Autodesk Inventor part; units mm, degrees
ref_plane "YZ Plane" through (0, 0, 0) normal (1, 0, 0) x (0, 1, 0)
ref_plane "XZ Plane" through (0, 0, 0) normal (0, 1, 0) x (-1, 0, 0)
ref_plane "XY Plane" through (0, 0, 0) normal (0, 0, 1) x (1, 0, 0)
sketch "Skizze3" plane through (0, 0, 0) normal (0, 0, 1) x (1, 0, 0)
  line L0 (0, 0) -> (-80, 0)
  line L1 (-80, 0) -> (-80, 100)
  line L2 (-80, 100) -> (0, 100)
  line L3 (0, 100) -> (0, 0)
  line L4 (-80, 100) -> (0, 100)
  line L5 (-40, 105.85) -> (-80, 105.85)
  line L6 (-80, 105.85) -> (-80, 100)
  line L7 (-80, 50) -> (-85.85, 50)
  line L8 (-85.85, 50) -> (-85.85, 98.2)
  line L9 (-85.85, 98.2) -> (-80, 98.2)
  line L10 (-80, 98.2) -> (-80, 50)
  line L11 (-40, 105.85) -> (-40, 100)
  dimension "d4" = 100
  dimension "d5" = 80
  dimension "d6" = 5.85
  dimension "d7" = 5.85
  dimension "d8" = 1.8
extrude "Extrusion3" add sketch "Skizze3" along normal blind 5 contours L0 L1 L2 L3
extrude "Extrusion4" add sketch "Skizze3" along normal blind 5 contours L7 L8 L9 L1 | L2 L6 L5 L11
fillet "Rundung1" radius 2 2 edges at (-85.85, 98.2, 2.5) (-80, 105.85, 2.5)
mirror "Spiegeln1" about plane through (-85.85, 50, 0) normal (0, -1, 0) of "Extrusion4", "Rundung1"
mirror "Spiegeln2" about plane through (-40, 0, 0) normal (1, 0, 0) of "Extrusion4", "Rundung1", "Spiegeln1"
fillet "Rundung2" radius 1.5 4 edges at (-80, 98.2, 2.5) (-80, 1.8, 2.5) (0, 1.8, 2.5) (0, 98.2, 2.5)
sketch "Skizze4" plane through (0, 0, 5) normal (0, 0, 1) x (1, 0, 0)
  circle A0 centre (-66.2696, 23.5053) radius 7.471
  point P0 (0, 0)
  point P1 (-74.5257, 11.4963)
  point P2 (-75.2763, 39.7173)
  point P3 (-61.9163, 37.7659)
  point P4 (-59.3644, 15.2491)
extrude "Extrusion5" cut sketch "Skizze4" against normal blind 10
equation "\"d7\" = d6"
properties part number "BT701_trajan20_21" material "Acryl"
CAD build for the part. Positions are in the model's coordinates, mm. A direction names the side the tool comes from. Round coordinates to 2 decimals unless told otherwise and drop trailing zeros. Write each loop counter-clockwise with the first axis right and the second up, starting at its lowest first coordinate (ties: lowest second). Pieces come first, ordered by that corner, then holes. Notation, with made-up numbers: (88.25, -34.5) -> (144.25, -34.5) arc R14 ccw to (144.25, -10.5) -> close; hole circle Ø4 at (-16.5, -5). An arc over 180 degrees is marked (long way). Answer in a Markdown table with one row per item. Add a question column.
Item 1: Drill centre lines: line 1 (X direction, y = 20.5, z = 2.65); line 2 (X direction, y = 20, z = 2.6); line 3 (X direction, y = 0.5, z = 1.75). Where is each one in solid material? Low to high. Write a range as from..to.
Item 2: Saw through at A-A, the plane z = 3.2. Write the cut outline in (x, y).
Item 3: Which spindle directions (+Z, -Z, +X, -X, +Y, -Y) get a long thin tool onto all of the face, cutting with end or side? Do faces 1 (the face through (0, -2, 2)), 2 (the face through (-83, 98.2, 2)), 3 (the face through (-41, -5.85, 2)), 4 (the face through (0, 102, 2)), 5 (the face through (-83, 1.8, 2)). Say none if no direction does.
Item 4: Drop flat-ended pins along their axis: pin 1 Ø2 at (y, z) = (101, 2.5) entering from +X; pin 2 Ø2 at (y, z) = (-2, 3) entering from -X; pin 3 Ø2.5 at (x, z) = (2, 1.5) entering from -Y; pin 4 Ø3 at (x, y) = (-22.5, 28) entering from -Z. Give the stop position or say it passes through.
Findings below:
| question | item | result |
|---|---|---|
| 1 | line 1 | x = -85.85..-73.11, -59.43..5.85 |
| 1 | line 2 | x = -85.85..-72.87, -59.67..5.85 |
| 1 | line 3 | x = -80.01..0.01 |
| 2 | outline | (-85.85, 3.8) arc R2 ccw to (-83.85, 1.8) -> (-81.5, 1.8) arc R1.5 cw to (-80, 0.3) -> (-80, -3.85) arc R2 ccw to (-78, -5.85) -> (-2, -5.85) arc R2 ccw to (0, -3.85) -> (0, 0.3) arc R1.5 cw to (1.5, 1.8) -> (3.85, 1.8) arc R2 ccw to (5.85, 3.8) -> (5.85, 96.2) arc R2 ccw to (3.85, 98.2) -> (1.5, 98.2) arc R1.5 cw to (0, 99.7) -> (0, 103.85) arc R2 ccw to (-2, 105.85) -> (-78, 105.85) arc R2 ccw to (-80, 103.85) -> (-80, 99.7) arc R1.5 cw to (-81.5, 98.2) -> (-83.85, 98.2) arc R2 ccw to (-85.85, 96.2) -> close; hole circle Ø14.94 at (-66.27, 23.51) |
| 3 | face 1 | +Z, -Z, +X, -Y |
| 3 | face 2 | +Z, -Z, -X, +Y |
| 3 | face 3 | +Z, -Z, +X, -X, -Y |
| 3 | face 4 | +Z, -Z, +X, +Y |
| 3 | face 5 | +Z, -Z, -X, -Y |
| 4 | pin 1 | stops at x = 0 |
| 4 | pin 2 | stops at x = -80 |
| 4 | pin 3 | stops at y = 1.6 |
| 4 | pin 4 | stops at z = 0 |
